The figure shows three views and two pictorial views of one solid part (mm, origin at its lowest corner). Answer the questions. Coordinates: 2 decimals unless noted, no trailing zeros. Order: outer loops, then holes, each group sorted by start corner. A loop starts at its lowest first (then second) coordinate and runs counter-clockwise, first axis right, second up.
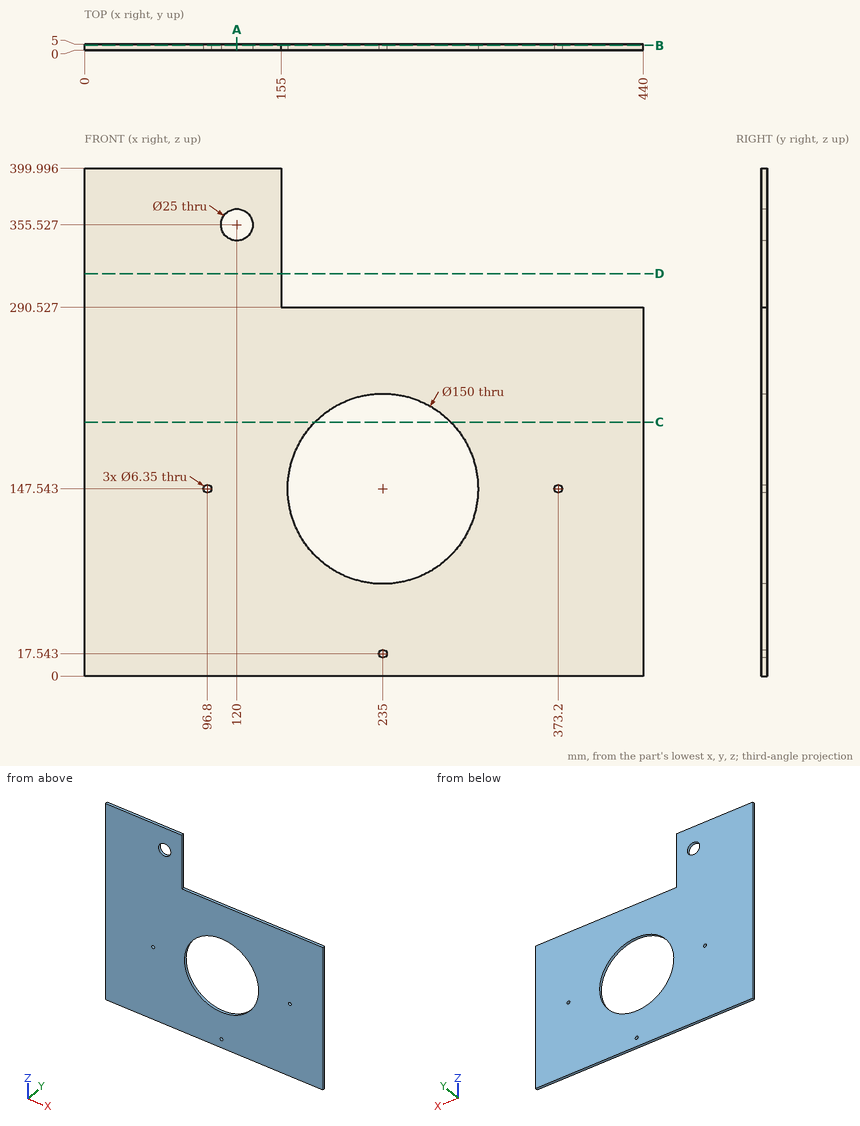
Q1. The part is cut by section C-C, the plane z = 200. Determine the outline of the cut face in (x, y).
Q2. The part is cut by section D-D, the plane z = 317. Determine the outline of the cut face in (x, y).
Q3. The part is cut by section B-B, the plane y = 3.95. State how many separate pieces and enclosed holes the cut face has, then the cut area to 3 significant figures.
Q4. The part is cut by section A-A, the plane x = 120. Determine the outline of the cut face in (y, z) (1 decimal).
Q5. Straight lines are drawn through the part: L1, parallel to Z at x = 373.2, y = 1.3; L2, parallel to Z at x = 236, y = 4.35; L3, parallel to Z at x = 399, y = 0.3. For each, find the intervals that lie inside material, in ascending order.
Q6. Each of these flat-tipped pins is pushed along its axis until it touches: P1, Ø1.5, axis at x = 323.5, y = 1.5, coming from the +Z side; P2, Ø5.5, axis at x = 235, z = 17.54, coming from the -Y side; P3, Ø1.5, axis at y = 3, z = 344, coming from the +X side. Where does it stop, or does it pass through?
Computed values:
1. outline: (0, 0) - (181.4, 0) - (181.4, 5) - (0, 5) - close; (288.6, 0) - (440, 0) - (440, 5) - (288.6, 5) - close
2. outline: (0, 0) - (155, 0) - (155, 5) - (0, 5) - close
3. separate pieces: 1
3. enclosed holes: 5
3. area: 127,000 mm2
4. outline: (0, 0) - (5, 0) - (5, 343) - (0, 343) - close; (0, 368) - (5, 368) - (5, 400) - (0, 400) - close
5. L1: z = 0 to 144.37, 150.72 to 290.53
5. L2: z = 0 to 14.53, 20.56 to 72.55, 222.54 to 290.53
5. L3: z = 0 to 290.53
6. P1: stops at z = 290.53
6. P2: passes through
6. P3: stops at x = 155
